from build123d import *

# Parameters (mm, degrees)
SZKIC1_W                        = 400
SZKIC1_H                        = 100
DODANIE_WYCI_GNI_CIE1_DEPTH     = 3
SZKIC_ZGI_CIA1_DEPTH            = 100
SZKIC_ZGI_CIA1_2_DEPTH          = 100
WYTNIJ_WYCI_GNI_CIE4_DEPTH      = 401.746800829
WYTNIJ_WYCI_GNI_CIE4_DEPTH_BACK = 401.746800829
SZKIC18_R                       = 5.5
WYTNIJ_WYCI_GNI_CIE5_DEPTH      = 383.009072614
WYTNIJ_WYCI_GNI_CIE5_DEPTH_BACK = 383.009072614
SZKIC19_R                       = 5.5
WYTNIJ_WYCI_GNI_CIE6_DEPTH      = 363.537857428
WYTNIJ_WYCI_GNI_CIE6_DEPTH_BACK = 363.537857428
SZKIC20_R                       = 5.5
SZKIC21_R                       = 5.5
WYTNIJ_WYCI_GNI_CIE7_DEPTH      = 10


# Read off the part's stored shape, not the designer's step: Szkic zgięcia1
with BuildPart() as part:
    # Szkic1 → Dodanie-wyciągnięcie1 (new body)
    with BuildSketch(Plane.XY):
        with Locations((200, 50)):
            Rectangle(SZKIC1_W, SZKIC1_H)
    extrude(amount=DODANIE_WYCI_GNI_CIE1_DEPTH)

    # Szkic zgięcia1 outline → Szkic zgięcia1 (cut)
    with BuildSketch(Plane(origin=(0, 0, 0), x_dir=(1, 0, 0), z_dir=(0, 1, 0))):
        with BuildLine():
            Line((0, -3), (144.331201036, -3))
            Line((144.331201036, -3), (146.51069296, -1.741669751))
            ThreePointArc((146.51069296, -1.741669751), (149.646045374, -0.442964258), (153.01069296, 0))
            Line((153.01069296, 0), (0, 0))
            Line((0, 0), (0, -3))
        make_face()
        with BuildLine():
            Line((253.48930704, -1.741669751), (255.668798964, -3))
            Line((255.668798964, -3), (400, -3))
            Line((400, -3), (400, 0))
            Line((400, 0), (246.98930704, 0))
            ThreePointArc((246.98930704, 0), (250.353954626, -0.442964258), (253.48930704, -1.741669751))
        make_face()
    extrude(amount=SZKIC_ZGI_CIA1_DEPTH, mode=Mode.SUBTRACT)

    # Szkic zgi_cia1 2 outline → Szkic zgi_cia1 2 (add)
    with BuildSketch(Plane(origin=(0, 0, 0), x_dir=(1, 0, 0), z_dir=(0, 1, 0))):
        with BuildLine():
            Line((20.714218978, -77.834399482), (148.01069296, -4.339745962))
            ThreePointArc((148.01069296, -4.339745962), (150.422502509, -3.340741737), (153.01069296, -3))
            Line((153.01069296, -3), (144.331201036, -3))
            Line((144.331201036, -3), (19.214218978, -75.236323271))
            Line((19.214218978, -75.236323271), (20.714218978, -77.834399482))
        make_face()
        with BuildLine():
            Line((255.668798964, -3), (246.98930704, -3))
            ThreePointArc((246.98930704, -3), (249.577497491, -3.340741737), (251.98930704, -4.339745962))
            Line((251.98930704, -4.339745962), (379.285781022, -77.834399482))
            Line((379.285781022, -77.834399482), (380.785781022, -75.236323271))
            Line((380.785781022, -75.236323271), (255.668798964, -3))
        make_face()
    extrude(amount=SZKIC_ZGI_CIA1_2_DEPTH)

    # Szkic18 → Wytnij-wyciągnięcie4 (cut, two sides: drawn at the far end of the back side and taken through both)
    with BuildSketch(Plane.XY.offset(3).offset(-WYTNIJ_WYCI_GNI_CIE4_DEPTH_BACK)):
        with Locations(Location((200.00069296, 49.999999995, 0), (0, 0, 180))):
            Circle(SZKIC18_R)
    extrude(amount=WYTNIJ_WYCI_GNI_CIE4_DEPTH + WYTNIJ_WYCI_GNI_CIE4_DEPTH_BACK, mode=Mode.SUBTRACT)

    # Szkic19 → Wytnij-wyciągnięcie5 (cut, two sides: drawn at the far end of the back side and taken through both)
    with BuildSketch(Plane(origin=(61.118161635, 0, -105.859761218), x_dir=(0.8660254037844382, 0, 0.500000000000001), z_dir=(-0.500000000000001, 0, 0.8660254037844382)).offset(-WYTNIJ_WYCI_GNI_CIE5_DEPTH_BACK)):
        with Locations(Location((250.39901436, 75, 0), (0, 0, 180))):
            Circle(SZKIC19_R)
        with Locations(Location((250.39901436, 25, 0), (0, 0, 180))):
            Circle(SZKIC19_R)
        with Locations(Location((317.3883214, 50, 0), (0, 0, 180))):
            Circle(SZKIC19_R)
        with Locations(Location((352.3883214, 50, 0), (0, 0, 180))):
            Circle(SZKIC19_R)
    extrude(amount=WYTNIJ_WYCI_GNI_CIE5_DEPTH + WYTNIJ_WYCI_GNI_CIE5_DEPTH_BACK, mode=Mode.SUBTRACT)

    # Szkic20 → Wytnij-wyciągnięcie6 (cut, two sides: drawn at the far end of the back side and taken through both)
    with BuildSketch(Plane(origin=(38.881838365, 0, 67.345319539), x_dir=(0.8660254037844382, 0, -0.500000000000001), z_dir=(0.500000000000001, 0, 0.8660254037844382)).offset(-WYTNIJ_WYCI_GNI_CIE6_DEPTH_BACK)):
        with Locations((96.011147154, 75)):
            Circle(SZKIC20_R)
        with Locations((96.011147154, 25)):
            Circle(SZKIC20_R)
        with Locations((29.021840113, 50)):
            Circle(SZKIC20_R)
    extrude(amount=WYTNIJ_WYCI_GNI_CIE6_DEPTH + WYTNIJ_WYCI_GNI_CIE6_DEPTH_BACK, mode=Mode.SUBTRACT)

    # Szkic21 → Wytnij-wyciągnięcie7 (cut)
    with BuildSketch(Plane(origin=(38.881838365, 0, 67.345319539), x_dir=(0.8660254037844382, 0, -0.500000000000001), z_dir=(0.500000000000001, 0, 0.8660254037844382))):
        with Locations((-5.978159887, 50)):
            Circle(SZKIC21_R)
    extrude(amount=-WYTNIJ_WYCI_GNI_CIE7_DEPTH, mode=Mode.SUBTRACT)


solid = part.part
Input: part model. Units: mm. Frame: model coordinates. A direction names the side the tool comes from. Coordinates: 2 decimals unless noted, no trailing zeros. Write each loop counter-clockwise with the first axis right and the second up, starting at its lowest first coordinate (ties: lowest second). Pieces come first, ordered by that corner, then holes. Notation, with made-up numbers: M 75,87.5 L 131,87.5 A24 cw 131,98.5 Z; hole C 64.25,36.25 d11. An arc over 180 degrees is marked long. Answer as a JSON object with one key per item and string values. Group by question number.
(1) Section B-B on z = 25.5. Output: boundary loops of the cut face in (x, y).
(2) Ray query, line 1 along Z through (x, y) = (220, 19); line 2 along X through (y, z) = (50, 1); line 3 along X through (y, z) = (91, 50.5). Return the intervals inside material, ascending. Write a range as [from, to].
(3) Section C-C on y = 6. Output: boundary loops of the cut face in (x, z), plus the area to 3 significant figures.
(4) Set-up query: faces 1 (the face through (120.649, 80.453, 18.381)), 2 (the face through (314.746, 49.3, 40.573)). Return all of +Z, -Z, +X, -X, +Y, -Y with unobstructed straight access to the full face (end or side cutting, diameter ignored); none if empty.
(5) Section D-D on x = 234. Output: boundary loops of the cut face in (y, z), plus the area to 3 significant figures.
(6) Mould query, pull axis X, two halves, no side actions, for faces 3 (the face through (189, 51, 0)), 4 (the face through (250.31, 49.3, 0.43)), 5 (the face through (83.471, 49.3, 41.602)), 6 (the face through (149.6, 49.3, 0.455)). Classes: pulls with the +X half, pulls with the -X half, needs draft (parallel to the pull), parting line crosses it, or undercut.
(7) Section A-A on y = 50. Give the number of separate pieces and of enclosed holes in the cut face, plus the area to 4 significant figures.
(8) Contact query for flat-ended pins moving along their axis: P1, Ø4, axis at x = 239.5, y = 36.5, coming from the +Z side; P2, Ø3, axis at y = 66, z = 62.5, coming from the +X side; P3, Ø4, axis at y = 37.5, z = 25.5, coming from the +X side. Output: stop coordinate, or through.
Result set:
{
 "1": {"outline": "M 105.36,0 L 111.36,0 L 111.36,100 L 105.36,100 Z; M 288.64,0 L 294.64,0 L 294.64,100 L 288.64,100 Z"},
 "2": {"line 1": "z = [0, 3]", "line 2": "x = [148.01, 194.5], [205.5, 251.99]", "line 3": "x = [62.06, 68.06], [331.94, 337.94]"},
 "3": {"outline": "M 19.21,75.24 L 146.51,1.74 A13 ccw 153.01,0 L 246.99,0 A13 ccw 253.49,1.74 L 380.79,75.24 L 379.29,77.83 L 251.99,4.34 A10 cw 246.99,3 L 153.01,3 A10 cw 148.01,4.34 L 20.71,77.83 Z", "area": "1,200 mm2"},
 "4": {"face 1": "none", "face 2": "+Z, +Y, -Y"},
 "5": {"outline": "M 0,0 L 100,0 L 100,3 L 0,3 Z", "area": "300 mm2"},
 "6": {"face 3": "needs draft", "face 4": "pulls with the +X half", "face 5": "undercut", "face 6": "pulls with the -X half"},
 "7": {"separate pieces": "6", "enclosed holes": "0", "area": "1,035 mm2"},
 "8": {"P1": "stops at z = 3", "P2": "stops at x = 361.32", "P3": "stops at x = 298.1"}
}
